from build123d import *

# Parameters (mm, degrees)
HOUSING_BOSS_EXTRUDE1_DEPTH           = 19.4
PLASTIC_SHEILDING_BOSS_EXTRUDE2_DEPTH = 16.7
SKETCH5_R                             = 1.75
MOUNTING_BRACKETS_BOSS_EXTRUDE3_DEPTH = 0.8
SKETCH6_R                             = 2.5
SHAFT_BOSS_EXTRUDE4_DEPTH             = 9.5
SHAFT_START                           = -6
SHAFT_EDGECUT_EXTRUDE1_DEPTH          = 6
CABLE_HOLE_CUT_EXTRUDE2_DEPTH         = 5


with BuildPart() as part:
    # Sketch2 → Housing Boss-Extrude1 (new body)
    with BuildSketch(Plane.XY):
        with BuildLine():
            Line((-6.1, -15.60119042), (0, -15.60119042))
            Line((0, -15.60119042), (6.1, -15.60119042))
            Line((6.1, -15.60119042), (6.1, -12.60119042))
            ThreePointArc((6.1, -12.60119042), (0, 14), (-6.1, -12.60119042))
            Line((-6.1, -12.60119042), (-6.1, -15.60119042))
        make_face()
    extrude(amount=-HOUSING_BOSS_EXTRUDE1_DEPTH)

    # Sketch4 → Plastic Sheilding Boss-Extrude2 (add)
    with BuildSketch(Plane.XY):
        with BuildLine():
            Line((0, -17.10119042), (-7.25, -17.10119042))
            Line((-7.25, -17.10119042), (-7.25, -14.253185025))
            Line((-7.25, -14.253185025), (-8.7, -13.245236981))
            Line((-8.7, -13.245236981), (-8.7, -10.968591523))
            ThreePointArc((-8.7, -10.968591523), (-7.444887158, -11.856376142), (-6.1, -12.60119042))
            Line((-6.1, -12.60119042), (-6.1, -15.60119042))
            Line((-6.1, -15.60119042), (6.1, -15.60119042))
            Line((6.1, -15.60119042), (6.1, -12.60119042))
            ThreePointArc((6.1, -12.60119042), (7.444887158, -11.856376142), (8.7, -10.968591523))
            Line((8.7, -10.968591523), (8.7, -13.245236981))
            Line((8.7, -13.245236981), (7.25, -14.253185025))
            Line((7.25, -14.253185025), (7.25, -17.10119042))
            Line((7.25, -17.10119042), (0, -17.10119042))
        make_face()
    extrude(amount=-PLASTIC_SHEILDING_BOSS_EXTRUDE2_DEPTH)

    # Sketch5 → Mounting Brackets Boss-Extrude3 (add)
    # profile 1 of 2: a face of its own
    with BuildSketch(Plane.XY):
        with BuildLine():
            Line((13.47442021, 3.8), (19.661172606, 1.480411881))
            ThreePointArc((19.661172606, 1.480411881), (21.285581553, 0.215191404), (21.9, -1.75))
            Line((21.9, -1.75), (20.4, -7.041502622))
            ThreePointArc((20.4, -7.041502622), (17.605339359, -10.428688818), (13.748967928, -8.328317944))
            Line((13.748967928, -8.328317944), (13.555441712, -3.5))
            ThreePointArc((13.555441712, -3.5), (13.999137791, 0.155374132), (13.47442021, 3.8))
        make_face()
        with Locations((18.45, -1.75)):
            Circle(SKETCH5_R, mode=Mode.SUBTRACT)
        with Locations((16.95, -7.041502622)):
            Circle(SKETCH5_R, mode=Mode.SUBTRACT)
    # profile 2 of 2: a face of its own
    with BuildSketch(Plane.XY):
        with BuildLine():
            Line((-13.748967928, -8.328317944), (-13.555441712, -3.5))
            ThreePointArc((-13.555441712, -3.5), (-13.999137791, 0.155374132), (-13.47442021, 3.8))
            Line((-13.47442021, 3.8), (-19.661172606, 1.480411881))
            ThreePointArc((-19.661172606, 1.480411881), (-21.285581553, 0.215191404), (-21.9, -1.75))
            Line((-21.9, -1.75), (-20.4, -7.041502622))
            ThreePointArc((-20.4, -7.041502622), (-17.605339359, -10.428688818), (-13.748967928, -8.328317944))
        make_face()
        with Locations(Location((-16.95, -7.041502622, 0), (0, 0, 180))):
            Circle(SKETCH5_R, mode=Mode.SUBTRACT)
        with Locations(Location((-18.45, -1.75, 0), (0, 0, 180))):
            Circle(SKETCH5_R, mode=Mode.SUBTRACT)
    extrude(amount=-MOUNTING_BRACKETS_BOSS_EXTRUDE3_DEPTH)

    # Sketch6 → Shaft Boss-Extrude4 (add)
    with BuildSketch(Plane.XY):
        with Locations((0, 8)):
            Circle(SKETCH6_R)
    extrude(amount=SHAFT_BOSS_EXTRUDE4_DEPTH)

    # Sketch7 → Shaft EdgeCut-Extrude1 (cut)
    with BuildSketch(Plane.XY.offset(9.5).offset(SHAFT_START)):
        with BuildLine():
            Line((-2, 9.5), (2, 9.5))
            ThreePointArc((2, 9.5), (0, 10.5), (-2, 9.5))
        make_face()
        with BuildLine():
            Line((-2, 6.5), (2, 6.5))
            ThreePointArc((2, 6.5), (0, 5.5), (-2, 6.5))
        make_face()
    extrude(amount=SHAFT_EDGECUT_EXTRUDE1_DEPTH, mode=Mode.SUBTRACT)

    # Sketch8 → Cable Hole Cut-Extrude2 (cut)
    with BuildSketch(Plane.XZ.offset(17.10119042)):
        Polygon((0, -2), (3.25, -2), (3.25, -3.2), (0, -3.2), (-3.25, -3.2), (-3.25, -2), align=None)
    extrude(amount=-CABLE_HOLE_CUT_EXTRUDE2_DEPTH, mode=Mode.SUBTRACT)


solid = part.part
Work out the finished part from the listing and answer in its coordinate system (mm). A direction names the side the tool comes from. Coordinates: 2 decimals unless noted, no trailing zeros. Write each loop counter-clockwise with the first axis right and the second up, starting at its lowest first coordinate (ties: lowest second). Pieces come first, ordered by that corner, then holes. Notation, with made-up numbers: M 46,-18 L 101,-18 A17 cw 101,-5 Z; hole C -14,48.25 d8. An arc over 180 degrees is marked long. Write item = value, one per line.
1. The part is cut by section A-A (z = -13). Determine the outline of the cut face in (x, y), then the cut area to 3 significant figures.
Solution:
outline = M -8.7,-13.25 L -7.25,-14.25 L -7.25,-17.1 L 7.25,-17.1 L 7.25,-14.25 L 8.7,-13.25 L 8.7,-10.97 A14 ccw long -8.7,-10.97 Z
area = 677 mm2
2. The part is cut by section B-B (x = 0). Determine the outline of the cut face in (y, z), then the cut area to 3 significant figures.
Solution:
outline = M -17.1,-16.7 L -15.6,-16.7 L -15.6,-19.4 L 14,-19.4 L 14,0 L 10.5,0 L 10.5,3.5 L 9.5,3.5 L 9.5,9.5 L 6.5,9.5 L 6.5,3.5 L 5.5,3.5 L 5.5,0 L -17.1,0 L -17.1,-2 L -12.1,-2 L -12.1,-3.2 L -17.1,-3.2 Z
area = 629 mm2
3. Flat-ended cylindrical pins translate along their axes: pin 1 (2 mm diameter, centred on x = 0.5, z = 6, fed in from -Y); pin 2 (0.8 mm diameter, centred on y = -14, z = -18.5, fed in from -X); pin 3 (10 mm diameter, centred on y = -11, z = -13, fed in from -X); pin 4 (1.1 mm diameter, centred on x = -0.5, y = 10, fed in from +Z). Find the tip coordinate at first contact, or state that the pin passes through.
Solution:
pin_1 = 6.5
pin_2 = -6.1
pin_3 = -12.65
pin_4 = 9.5
4. The part is cut by section C-C (z = 1). Determine the outline of the cut face in (x, y), then the cut area to 3 significant figures.
Solution:
outline = C 0,8 d5
area = 19.6 mm2
5. For faces 1 (the face through (2.385, 8.751, 3.628)), 2 (the face through (0, -15, -3.2)), 3 (the face through (0, 10, 3.5)), 4 (the face through (0, 6, 3.5)), determine the directions among +Z, -Z, +X, -X, +Y, -Y from which every point of the face is accessible in a straight line to the end or side of a thin tool.
Solution:
face_1 = +Z
face_2 = -Y
face_3 = +Z, +X, -X, +Y
face_4 = +Z, +X, -X, -Y
6. Straight lines are drawn through the part: line 1 (Y direction, x = -16.95, z = -0.2); line 2 (Y direction, x = -18.45, z = -0.3); line 3 (Z direction, x = 4.5, y = 7). For each, find the intervals that lie inside material, in ascending order. Write a range as from..to.
Solution:
line_1 = -10.49..-8.79, -5.29..-2.65, -0.85..2.5
line_2 = -10.15..-7.94, -6.14..-3.5, 0..1.93
line_3 = -19.4..0
7. Determine the mould class of faces 5 (the face through (18.62, -6.52, -0.39)), 6 (the face through (-17.671, -10.415, -0.394)), 7 (the face through (8.7, -12, -8)), 8 (the face through (0, 9.5, 6)) for opening direction X: released by +X, released by -X, zero draft, split by the parting line, or undercut.
Solution:
face_5 = undercut
face_6 = undercut
face_7 = released by +X
face_8 = zero draft
8. The part is cut by section D-D (z = 6.5). Determine the outline of the cut face in (x, y), then the cut area to 3 significant figures.
Solution:
outline = M -2,6.5 L 2,6.5 A2.5 ccw 2,9.5 L -2,9.5 A2.5 ccw Z
area = 14.0 mm2
